Check sheet for the modelled part. Datum: model origin and axes. Units: mm. A direction names the side the tool comes from. Round coordinates to 2 decimals unless told otherwise and drop trailing zeros. Loops run counter-clockwise (first coordinate to the right, second up) from the corner with the lowest first, then second, coordinate; pieces in that order, holes last. Notation, with made-up numbers: (63, 82) -> (89, 82) arc R19 ccw to (89, 95) -> close; hole circle Ø5 at (5, 50.25). An arc over 180 degrees is marked (long way). One line per item, written item: value. Start each with the question number.
1. Cross-section at A-A on x = 0. Record the cut outline in (y, z).
2. Cross-section at C-C on z = 35.5. Record the cut outline in (x, y), then the cut area to 3 significant figures.
3. Material ranges on L1, parallel to Z at x = -6.75, y = 0.6; L2, parallel to X at y = -0.9, z = 13; L3, parallel to X at y = 0, z = 9, recorded low to high.
4. Cross-section at D-D on z = 18. Record the cut outline in (x, y).
5. Release check for a two-part mould opening along X. For faces 3 (the face through (10.18, 0.01, -5.35)), 4 (the face through (-4.29, 0.01, 43.19)), 5 (the face through (-11.156, 0.014, -4.869)) record: +X half, -X half, draft (parallel to the pull), parting line (faces both ways), or undercut.
6. Set-up check for faces 1 (the face through (-9.44, 0.01, 33.89)), 2 (the face through (-7.254, 0.014, -8.925)): record each of +Z, -Z, +X, -X, +Y, -Y from which the full face is reachable in a straight line by a thin tool's end or side.
7. Go/stop test with a flat-tipped pin: pin 1 (1 mm diameter, centred on y = -1, z = 27, fed in from -X). Record where the tip stops, or that it passes through.
8. Cross-section at B-B on y = -0.05. Record the cut outline in (x, z).
from build123d import *

# Parameters (mm, degrees)
SKETCH1_R           = 1.5
BOSS_EXTRUDE3_DEPTH = 1
BOSS_EXTRUDE5_DEPTH = 1


with BuildPart() as part:
    # Sketch1 → Boss-Extrude3 (new, symmetric)
    with BuildSketch(Plane(origin=(0, 0, 0), x_dir=(1, 0, 0), z_dir=(0, 1, 0))):
        with BuildLine():
            Line((10.514574075, -4.657653059), (11.5, 0))
            ThreePointArc((11.5, 0), (11.485144533, -0.58434155), (11.440616514, -1.167173419))
            ThreePointArc((11.440616514, -1.167173419), (12.15387442, 0.169569159), (13.599672235, 0.622654405))
            ThreePointArc((13.599672235, 0.622654405), (15.211699124, 2.97560242), (12.831884171, 4.547695243))
            ThreePointArc((12.831884171, 4.547695243), (10.157548748, 5.392050021), (10.95665555, 8.080252631))
            ThreePointArc((10.95665555, 8.080252631), (10.987967437, 10.932272023), (8.135825754, 10.91545339))
            ThreePointArc((8.135825754, 10.91545339), (5.443597104, 10.130017304), (4.612843157, 12.808608879))
            ThreePointArc((4.612843157, 12.808608879), (3.052863924, 15.196381867), (0.691754597, 13.596332557))
            ThreePointArc((0.691754597, 13.596332557), (-1.109021523, 11.446399926), (-3.289035023, 13.210640864))
            ThreePointArc((-3.289035023, 13.210640864), (-5.913396009, 14.327656739), (-6.985968373, 11.684820465))
            ThreePointArc((-6.985968373, 11.684820465), (-7.287049374, 8.896567395), (-10.079986001, 9.150555482))
            ThreePointArc((-10.079986001, 9.150555482), (-12.882306434, 8.619523243), (-12.304062381, 5.826562651))
            ThreePointArc((-12.304062381, 5.826562651), (-11.145420085, 4.850260698), (-11.003753067, 3.341768759))
            ThreePointArc((-11.003753067, 3.341768759), (-4.007182474, -10.77926197), (10.514574075, -4.657653059))
        make_face()
        with Locations(Location((0, 0, 0), (0, 0, 270))):
            Circle(SKETCH1_R, mode=Mode.SUBTRACT)
    extrude(amount=BOSS_EXTRUDE3_DEPTH, both=True)

    # Sketch1<5> → Boss-Extrude5 (add, symmetric)
    with BuildSketch(Plane(origin=(0, 0, 0), x_dir=(1, 0, 0), z_dir=(0, 1, 0))):
        with BuildLine():
            Line((2.806807826, -41.088702969), (10.514574075, -4.657653059))
            ThreePointArc((10.514574075, -4.657653059), (1.846708509, -11.35075626), (-8.495825279, -7.750545324))
            ThreePointArc((-8.495825279, -7.750545324), (-7.347088724, -15.263704681), (-7.738414168, -22.854094893))
            Line((-7.738414168, -22.854094893), (-11.192007229, -45.231550072))
            Line((-11.192007229, -45.231550072), (2.806807826, -41.088702969))
        make_face()
    extrude(amount=BOSS_EXTRUDE5_DEPTH, both=True)


solid = part.part
Taken from the geometry:
1. outline: (-1, -11.92) -> (1, -11.92) -> (1, -1.5) -> (-1, -1.5) -> close; (-1, 1.5) -> (1, 1.5) -> (1, 41.92) -> (-1, 41.92) -> close
2. outline: (-9.69, -1) -> (3.99, -1) -> (3.99, 1) -> (-9.69, 1) -> close
2. area: 27.4 mm2
3. L1: z = -13.68 to -11.31, -9.58 to 43.92
3. L2: x = -7.53 to 8.75
3. L3: x = -8.2 to 9.6
4. outline: (-7.31, -1) -> (7.69, -1) -> (7.69, 1) -> (-7.31, 1) -> close
5. face 3: undercut
5. face 4: +X half
5. face 5: -X half
6. face 1: -X, +Y, -Y
6. face 2: +Y, -Y
7. pin 1: stops at x = -8.46
8. outline: (-12.3, -5.83) arc R2 ccw (long way) to (-10.08, -9.15) arc R2 cw to (-6.99, -11.68) arc R2 ccw (long way) to (-3.29, -13.21) arc R2 cw to (0.69, -13.6) arc R2 ccw (long way) to (4.61, -12.81) arc R2 cw to (8.14, -10.92) arc R2 ccw (long way) to (10.96, -8.08) arc R2 cw to (12.83, -4.55) arc R2 ccw (long way) to (13.6, -0.62) arc R2 cw to (11.44, 1.17) arc R11.5 cw to (11.5, 0) -> (2.81, 41.09) -> (-11.19, 45.23) -> (-7.74, 22.85) arc R37.46 cw to (-8.5, 7.75) arc R11.5 ccw to (-11, -3.34) arc R2 cw to start; hole circle Ø3 at (0, 0)
